Build history of the part. All positions in model axes, mm. A direction names the side the tool comes from. Coordinates: 2 decimals unless noted, no trailing zeros. Loops run counter-clockwise (first coordinate to the right, second up) from the corner with the lowest first, then second, coordinate; pieces in that order, holes last. Notation, with made-up numbers: (73.25, -17) - (90.25, -17) arc R7 cw to (90.25, -5) - close; hole circle Ø6 at (54.5, 45.5). An arc over 180 degrees is marked (long way). One line per item, written item: value.
```python
from build123d import *

# Parameters (mm, degrees)
PAD_DEPTH             = 2
PCB_SKETCH_F9E005_R   = 3
PCB_SKETCH_F9E005_R_2 = 1.65
PAD003_DEPTH          = 3.3
SKETCH_W              = 21
SKETCH_H              = 28
PAD015_DEPTH          = 1.6
SKETCH017_R           = 7
SKETCH017_R_2         = 3.9
PAD016_DEPTH          = 6.5


with BuildPart() as part:
    # PCB_Sketch_f9e4 → Pad (new body)
    with BuildSketch(Plane.ZY):
        with BuildLine():
            Line((48.934205, 15.25), (77.594554, 15.25))
            ThreePointArc((77.594554, 15.25), (77.970292, 15.176729), (78.290965, 14.967643))
            Line((78.290965, 14.967643), (88.036374, 7.842738))
            ThreePointArc((88.626567, 7.65), (88.316134, 7.699405), (88.036374, 7.842738))
            Line((125, 7.65), (88.626567, 7.65))
            ThreePointArc((126, 8.65), (125.707107, 7.942893), (125, 7.65))
            Line((126, 8.65), (126, 45.95))
            Line((126, 45.95), (126, 46.85))
            ThreePointArc((125, 47.85), (125.707107, 47.557107), (126, 46.85))
            Line((104.561886, 47.85), (125, 47.85))
            ThreePointArc((104.438586, 47.842369), (104.500118, 47.84809), (104.561886, 47.85))
            Line((104.438586, 47.842369), (27.548891, 38.288977))
            ThreePointArc((27.250327, 38.20537), (27.396349, 38.258815), (27.548891, 38.288977))
            Line((27.250327, 38.20537), (0.583058, 26.017458))
            ThreePointArc((0, 25.108525), (0.158304, 25.648452), (0.583058, 26.017458))
            Line((0, 25.108525), (0, 1))
            ThreePointArc((1, 0), (0.292893, 0.292893), (0, 1))
            Line((1, 0), (33.815795, 0))
            ThreePointArc((34.546452, 0.317255), (34.214075, 0.082738), (33.815795, 0))
            Line((34.546452, 0.317255), (48.203548, 14.932745))
            ThreePointArc((48.203548, 14.932745), (48.535925, 15.167262), (48.934205, 15.25))
        make_face()
    extrude(amount=PAD_DEPTH)

    # PCB_Sketch_f9e005 (on Face21 of Pad) → Pad003 (join)
    with BuildSketch(Plane.ZY.offset(2)):
        with Locations((4.15, 23.166726)):
            Circle(PCB_SKETCH_F9E005_R)
        with Locations((4.15, 23.166726)):
            Circle(PCB_SKETCH_F9E005_R_2, mode=Mode.SUBTRACT)
        with Locations((4.15, 4.65)):
            Circle(PCB_SKETCH_F9E005_R)
        with Locations((4.15, 4.65)):
            Circle(PCB_SKETCH_F9E005_R_2, mode=Mode.SUBTRACT)
        with Locations((95.5, 43.35)):
            Circle(PCB_SKETCH_F9E005_R)
        with Locations((95.5, 43.35)):
            Circle(PCB_SKETCH_F9E005_R_2, mode=Mode.SUBTRACT)
        with Locations((99.833274, 10.683274)):
            Circle(PCB_SKETCH_F9E005_R)
        with Locations((99.833274, 10.683274)):
            Circle(PCB_SKETCH_F9E005_R_2, mode=Mode.SUBTRACT)
    extrude(amount=PAD003_DEPTH)

    # Sketch → Pad015 (join)
    with BuildSketch(Plane.XY):
        with Locations((10.5, 14)):
            Rectangle(SKETCH_W, SKETCH_H)
    extrude(amount=PAD015_DEPTH)

    # Sketch017 (on Face4 of Pad015) → Pad016 (join)
    with BuildSketch(Plane(origin=(0, 0, 0), x_dir=(0, 0, 1), z_dir=(1, 0, 0))):
        with Locations((66.139557, -28.292141)):
            Circle(SKETCH017_R)
        with Locations((66.139557, -28.292141)):
            Circle(SKETCH017_R_2, mode=Mode.SUBTRACT)
    extrude(amount=PAD016_DEPTH)


solid = part.part
```
Item 1: Cut at D-D, the plane z = 95.5. Write the cut outline in (x, y).
Check result:
outline: (-5.3, 40.35) - (-2, 40.35) - (-2, 7.65) - (0, 7.65) - (0, 46.73) - (-2, 46.73) - (-2, 46.35) - (-5.3, 46.35) - (-5.3, 45) - (-2, 45) - (-2, 41.7) - (-5.3, 41.7) - close
Item 2: Pull direction Y, two halves, no side cores. Call faces 1 (the face through (-0.986, 43.133, 66.532)), 2 (the face through (-5.3, 42, 97)), 3 (the face through (-2, 23, 4)): released by +Y, released by -Y, zero draft, split by the parting line, or undercut.
Check result:
face 1: released by +Y
face 2: zero draft
face 3: undercut
Item 3: Cut at A-A, the plane z = 4.15. Write the cut outline in (x, y).
Check result:
outline: (-5.3, 1.65) - (-2, 1.65) - (-2, 0) - (0, 0) - (0, 27.65) - (-2, 27.65) - (-2, 26.17) - (-5.3, 26.17) - (-5.3, 24.82) - (-2, 24.82) - (-2, 21.52) - (-5.3, 21.52) - (-5.3, 20.17) - (-2, 20.17) - (-2, 7.65) - (-5.3, 7.65) - (-5.3, 6.3) - (-2, 6.3) - (-2, 3) - (-5.3, 3) - close
Item 4: Cut at B-B, the plane x = 18.5. Write the cut outline in (y, z), then the cut area to 3 significant figures.
Check result:
outline: (0, 0) - (28, 0) - (28, 1.6) - (0, 1.6) - close
area: 44.8 mm^2
Item 5: Probe probe 1 along Y at (x, z) = (-3.3, 4.15); probe 2 along X at (y, z) = (36, 42.5); probe 3 along Z at (x, y) = (-2.5, 23.5). List the from-to ranges inside material, lowest first. Write a range as from..to.
Check result:
probe 1: y = 1.65..3, 6.3..7.65, 20.17..21.52, 24.82..26.17
probe 2: x = -2..0
probe 3: z = 1.17..2.53, 5.77..7.13
Item 6: Tool access for faces 4 (the face through (-2, 5, 4)), 5 (the face through (3.2, 27.12, 69.86)), 6 (the face through (-0.986, 7.523, 41.279)), 7 (the face through (-5.3, 9, 101)): list every direction of +Z, -Z, +X, -X, +Y, -Y with a clear straight run to the whole face (end or side of a thin tool).
Check result:
face 4: -X
face 5: +X
face 6: +X, -X, -Y
face 7: +Z, -Z, -X, +Y, -Y
Item 7: Cut at C-C, the plane y = 43.35. Write the cut outline in (x, z).
Check result:
outline: (-5.3, 92.5) - (-2, 92.5) - (-2, 68.28) - (0, 68.28) - (0, 126) - (-2, 126) - (-2, 98.5) - (-5.3, 98.5) - (-5.3, 97.15) - (-2, 97.15) - (-2, 93.85) - (-5.3, 93.85) - close
Item 8: Drop flat-ended pins along their axis: P1, Ø1.8, axis at x = 15, z = 0.5, coming from the +Y side; P2, Ø7, axis at y = 27, z = 66.5, coming from the +X side; P3, Ø5, axis at x = 4.5, y = 42, coming from the +Z side; P4, Ø10, axis at x = -1.5, z = 51.5, coming from the -Y side. Give the stop position or say it passes through.
Check result:
P1: stops at y = 28
P2: stops at x = 6.5
P3: passes through
P4: stops at y = 13.11
